Check sheet for the modelled part. Datum: model origin and axes. Units: mm. Face numbers are marked on the shaded views. A direction names the side the tool comes from. Round coordinates to 2 decimals unless told otherwise and drop trailing zeros. Write each loop counter-clockwise with the first axis right and the second up, starting at its lowest first coordinate (ties: lowest second). Pieces come first, ordered by that corner, then holes. Notation, with made-up numbers: (-31.5, 4) -> (6.5, 4) arc R31 ccw to (6.5, 41) -> close; hole circle Ø6 at (12.25, 44). An arc over 180 degrees is marked (long way). Use one line per item in the form item = value. Start each with the question number.
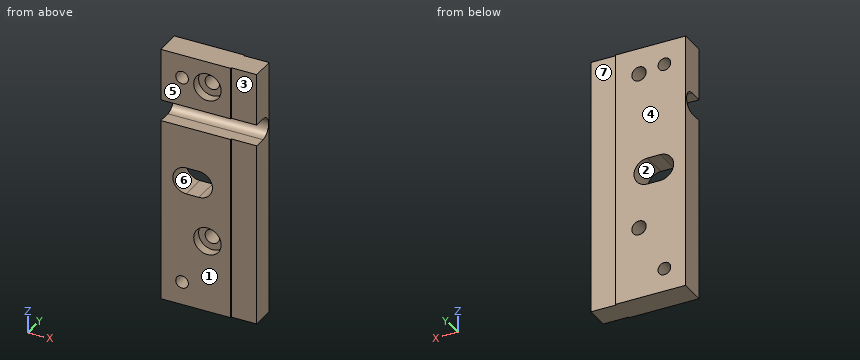
```python
from build123d import *

# Parameters (mm, degrees)
SKETCH1_W                                        = 61
SKETCH1_H                                        = 6.1
BOSS_EXTRUDE1_DEPTH                              = 22.5
SKETCH2_OUTSIDE_W                                = 76.06
SKETCH2_OUTSIDE_H                                = 21.16
SKETCH2_OUTSIDE_W_2                              = 61
SKETCH2_OUTSIDE_H_2                              = 5.55
CUT_EXTRUDE1_DEPTH                               = 6
CUT_EXTRUDE3_DEPTH                               = 23.5
CUT_EXTRUDE4_DEPTH                               = 7.1
SKETCH7_R                                        = 1.5
CUT_EXTRUDE5_DEPTH                               = 7.1
CBORE_FOR_M3_PAN_HEAD_MACHINE_SCREW2_D           = 3.4
CBORE_FOR_M3_PAN_HEAD_MACHINE_SCREW2_CBORE_D     = 6.5
CBORE_FOR_M3_PAN_HEAD_MACHINE_SCREW2_CBORE_DEPTH = 2.2


with BuildPart() as part:
    # Sketch1 → Boss-Extrude1 (new body)
    with BuildSketch(Plane(origin=(0, 0, 0), x_dir=(0, 0, -1), z_dir=(1, 0, 0))):
        with Locations((30.5, 0)):
            Rectangle(SKETCH1_W, SKETCH1_H)
    extrude(amount=BOSS_EXTRUDE1_DEPTH)

    # Sketch2 outside → Cut-Extrude1 (cut)
    with BuildSketch(Plane(origin=(22.5, 0, 0), x_dir=(0, 0, -1), z_dir=(1, 0, 0))):
        with Locations((30.5, 0)):
            Rectangle(SKETCH2_OUTSIDE_W, SKETCH2_OUTSIDE_H)
        with Locations((30.5, 0)):
            Rectangle(SKETCH2_OUTSIDE_W_2, SKETCH2_OUTSIDE_H_2, mode=Mode.SUBTRACT)
    extrude(amount=-CUT_EXTRUDE1_DEPTH, mode=Mode.SUBTRACT)

    # Sketch5 → Cut-Extrude3 (cut, through all)
    with BuildSketch(Plane.ZY):
        with BuildLine():
            Line((-12.3486, 0.0496), (-12.3486, -3.05))
            Line((-12.3486, -3.05), (-17.4134, -3.05))
            Line((-17.4134, -3.05), (-17.4134, 0.0496))
            ThreePointArc((-17.4134, 0.0496), (-14.881, 2.582), (-12.3486, 0.0496))
        make_face()
    extrude(amount=-CUT_EXTRUDE3_DEPTH, mode=Mode.SUBTRACT)

    # Sketch6 → Cut-Extrude4 (cut, through all)
    with BuildSketch(Plane(origin=(0, 3.05, 0), x_dir=(1, 0, 0), z_dir=(0, 1, 0))):
        with BuildLine():
            Line((9, 27.325), (6, 27.325))
            ThreePointArc((6, 27.325), (2.825, 30.5), (6, 33.675))
            Line((6, 33.675), (9, 33.675))
            ThreePointArc((9, 33.675), (12.175, 30.5), (9, 27.325))
        make_face()
    extrude(amount=-CUT_EXTRUDE4_DEPTH, mode=Mode.SUBTRACT)

    # Sketch7 → Cut-Extrude5 (cut, through all)
    with BuildSketch(Plane(origin=(0, 3.05, 0), x_dir=(1, 0, 0), z_dir=(0, 1, 0))):
        with Locations(Location((5, 55.5, 0), (0, 0, 270))):  # turned: the seam where the file's is
            Circle(SKETCH7_R)
        with Locations(Location((5, 5.5, 0), (0, 0, 270))):  # turned: the seam where the file's is
            Circle(SKETCH7_R)
    extrude(amount=-CUT_EXTRUDE5_DEPTH, mode=Mode.SUBTRACT)

    # CBORE for M3 Pan Head Machine Screw2 (through all)
    with Locations(Plane(origin=(0, -3.05, 0), x_dir=(-1, 0, 0), z_dir=(0, -1, 0))):
        with Locations((-11, 6.175), (-11, 43.85)):
            CounterBoreHole(CBORE_FOR_M3_PAN_HEAD_MACHINE_SCREW2_D / 2, CBORE_FOR_M3_PAN_HEAD_MACHINE_SCREW2_CBORE_D / 2, CBORE_FOR_M3_PAN_HEAD_MACHINE_SCREW2_CBORE_DEPTH)


solid = part.part
```
1. Scan lines: probe 1 along Z at (x, y) = (11, -1.8) (3 decimals); probe 2 along Z at (x, y) = (5.75, 0.75); probe 3 along Y at (x, z) = (9.75, -4). Record each from-to range of solid material in increasing order.
2. Mould release check, pull along X, two halves, no side actions. Record for the marked faces 1 and 2: +X half, -X half, draft (parallel to the pull), parting line (faces both ways), or undercut.
3. Sectioned sample at A-A (z = -43.85). Enter the section's corners in (x, y) (3 decimals), and give its area (3 significant figures).
4. Tool access check on the marked faces 3, 4, 5, 6 and 7. Record the directions out of +Z, -Z, +X, -X, +Y, -Y that give a thin tool (end or side, any length) a straight path to the whole face; none if there is none.
5. Sectioned sample at B-B (x = 11). Enter the section's corners in (y, z) (3 decimals), and give its area (3 significant figures).
6. Depth check by flat-ended pin: pin 1 (1.8 mm diameter, centred on x = 18.5, z = -5.5, fed in from -Y) (3 decimals); pin 2 (5 mm diameter, centred on x = 19.5, z = -30, fed in from +Y) (3 decimals). Enter the tip coordinate at first touch or a pass-through.
7. Sectioned sample at C-C (y = 1.25). Enter the section's corners in (x, z) (3 decimals), and give its area (3 significant figures).
8. Sectioned sample at D-D (x = 20.5). Enter the section's corners in (y, z) (3 decimals), and give its area (3 significant figures).
Returned:
q1.probe_1 = -61 to -47.1, -40.6 to -32.966, -28.034 to -17.413, -12.349 to -9.425, -2.925 to 0
q1.probe_2 = -61 to -56.8, -54.2 to -33.67, -27.33 to -17.31, -12.45 to -6.8, -4.2 to 0
q1.probe_3 = -0.85 to 3.05
q2.face_1 = draft
q2.face_2 = undercut
q3.outline = (0, -3.05) -> (7.75, -3.05) -> (7.75, -0.85) -> (9.3, -0.85) -> (9.3, 3.05) -> (0, 3.05) -> close; (12.7, -0.85) -> (14.25, -0.85) -> (14.25, -3.05) -> (16.5, -3.05) -> (16.5, -2.775) -> (22.5, -2.775) -> (22.5, 2.775) -> (16.5, 2.775) -> (16.5, 3.05) -> (12.7, 3.05) -> close
q3.area = 106 mm^2
q4.face_3 = +Z, -Z, +X, -Y
q4.face_4 = +Z, -Z, +X, -X, +Y
q4.face_5 = +Z, -Z, +X, -X, -Y
q4.face_6 = +Y, -Y
q4.face_7 = +Z, -Z, +X, +Y
q5.outline = (-3.05, -61) -> (3.05, -61) -> (3.05, -45.55) -> (-0.85, -45.55) -> (-0.85, -47.1) -> (-3.05, -47.1) -> close; (-3.05, -40.6) -> (-0.85, -40.6) -> (-0.85, -42.15) -> (3.05, -42.15) -> (3.05, -32.966) -> (-3.05, -32.966) -> close; (-3.05, -28.034) -> (3.05, -28.034) -> (3.05, -7.875) -> (-0.85, -7.875) -> (-0.85, -9.425) -> (-3.05, -9.425) -> (-3.05, -12.349) -> (0.05, -12.349) arc R2.532 cw to (0.05, -17.413) -> (-3.05, -17.413) -> close; (-3.05, -2.925) -> (-0.85, -2.925) -> (-0.85, -4.475) -> (3.05, -4.475) -> (3.05, 0) -> (-3.05, 0) -> close
q5.area = 261 mm^2
q6.pin_1 = -2.775
q6.pin_2 = 2.775
q7.outline = (0, -61) -> (22.5, -61) -> (22.5, -17.111) -> (0, -17.111) -> close; (0, -12.651) -> (22.5, -12.651) -> (22.5, 0) -> (0, 0) -> close; hole circle Ø3 at (5, -55.5); hole circle Ø3 at (5, -5.5); hole (6, -33.675) -> (9, -33.675) arc R3.175 ccw to (9, -27.325) -> (6, -27.325) arc R3.175 ccw to start; hole circle Ø3.4 at (11, -43.85); hole circle Ø3.4 at (11, -6.175)
q7.area = 1,190 mm^2
q8.outline = (-2.775, -61) -> (2.775, -61) -> (2.775, 0) -> (-2.775, 0) -> (-2.775, -12.349) -> (0.05, -12.349) arc R2.532 cw to (0.05, -17.413) -> (-2.775, -17.413) -> close
q8.area = 314 mm^2
